Here's the drawing with two shaded views (mm, measured from the low corner). I have some questions. Coordinates: 2 decimals unless noted, no trailing zeros. Order: outer loops, then holes, each group sorted by start corner. A loop starts at its lowest first (then second) coordinate and runs counter-clockwise, first axis right, second up. Notation, with made-up numbers: (17.5, 55) -> (45.5, 55) arc R15 cw to (45.5, 76) -> close; hole circle Ø5 at (45.25, 44.25). An arc over 180 degrees is marked (long way). Answer as a JSON object with one key per item and string values. Group by question number.
(1) I want a section at D-D, the plane x = 1064. List the corners of the cut face in (y, z) for me, plus the area to 3 significant figures.
(2) I need wall thicknesses on line 1 (X direction, y = 702, z = 890); line 2 (Z direction, x = 276.5, y = 467.5); line 3 (Y direction, x = 227, z = 895). Which ranges of each line are inside material? Lowest first, please.
(3) If we mould it in two halves opening along Y, with no side actions, what happens to the marked faces 1, 2, 3 and 4? For each: pulls with the +Y half, pulls with the -Y half, needs draft (parallel to the pull), parting line crosses it, or undercut.
(4) I want a section at B-B, the plane y = 49.5. List the corners of the cut face in (x, z) for me, plus the area to 3 significant figures.
(5) For pin 1 (4 mm diameter, centred on x = 616, y = 247, fed in from -Z), with a flat end and sliding along its axis, tell me the tip position at first contact or that it passes through.
(6) I want a section at C-C, the plane z = 504.5. List the corners of the cut face in (x, y) for me.
(7) I want a section at A-A, the plane z = 849. List the corners of the cut face in (x, y) for me.
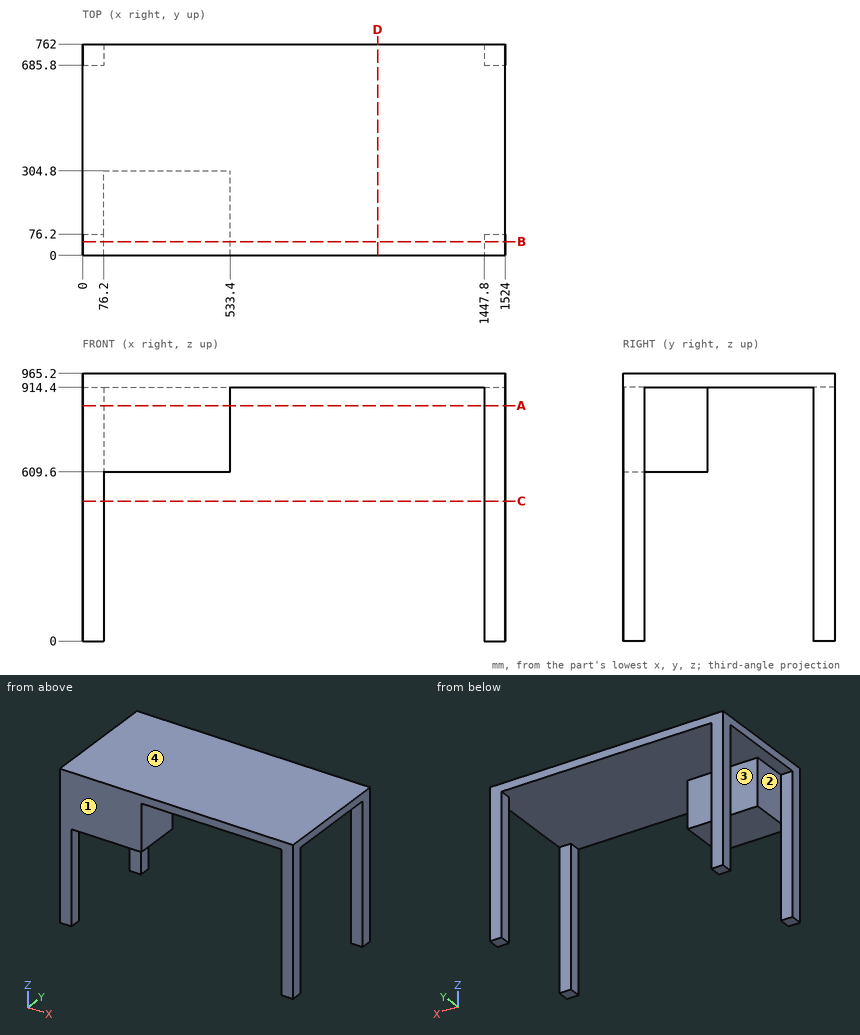
Computed values:
{
 "1": {"outline": "(0, 914.4) -> (762, 914.4) -> (762, 965.2) -> (0, 965.2) -> close", "area": "38,700 mm2"},
 "2": {"line 1": "x = 0 to 76.2, 1447.8 to 1524", "line 2": "z = 914.4 to 965.2", "line 3": "y = 0 to 304.8"},
 "3": {"face 1": "pulls with the -Y half", "face 2": "undercut", "face 3": "pulls with the +Y half", "face 4": "needs draft"},
 "4": {"outline": "(0, 0) -> (76.2, 0) -> (76.2, 609.6) -> (533.4, 609.6) -> (533.4, 914.4) -> (1447.8, 914.4) -> (1447.8, 0) -> (1524, 0) -> (1524, 965.2) -> (0, 965.2) -> close", "area": "356,000 mm2"},
 "5": {"pin 1": "stops at z = 914.4"},
 "6": {"outline": "(0, 0) -> (76.2, 0) -> (76.2, 76.2) -> (0, 76.2) -> close; (0, 685.8) -> (76.2, 685.8) -> (76.2, 762) -> (0, 762) -> close; (1447.8, 0) -> (1524, 0) -> (1524, 76.2) -> (1447.8, 76.2) -> close; (1447.8, 685.8) -> (1524, 685.8) -> (1524, 762) -> (1447.8, 762) -> close"},
 "7": {"outline": "(0, 0) -> (533.4, 0) -> (533.4, 304.8) -> (76.2, 304.8) -> (76.2, 76.2) -> (0, 76.2) -> close; (0, 685.8) -> (76.2, 685.8) -> (76.2, 762) -> (0, 762) -> close; (1447.8, 0) -> (1524, 0) -> (1524, 76.2) -> (1447.8, 76.2) -> close; (1447.8, 685.8) -> (1524, 685.8) -> (1524, 762) -> (1447.8, 762) -> close"}
}
